```python
from build123d import *

# Parameters (mm, degrees)
BOSS_EXTRUDE1_DEPTH = 4
FILLET1_R           = 4
CHAMFER1_SIZE       = 3
CHAMFER2_SIZE       = 5
FILLET2_R           = 4
SKETCH2_R           = 1.6
CUT_EXTRUDE1_DEPTH  = 142.477913471
CUT_EXTRUDE2_DEPTH  = 2
FILLET3_R           = 3
SKETCH4_R           = 1.6
CUT_EXTRUDE3_DEPTH  = 142.477913471


with BuildPart() as part:
    # Sketch1 → Boss-Extrude1 (new body)
    with BuildSketch(Plane.XY):
        Polygon((-12, -87.8), (12, -87.8), (12, -56.4), (20, -56.4), (20, -95.8), (0, -115.8), (0, -140), (-20, -140), (-20, -95.8), align=None)
    extrude(amount=BOSS_EXTRUDE1_DEPTH)

    # Fillet1
    fillet1_edges = [part.edges().sort_by_distance(p)[0] for p in [
        (12, -56.4, 2),
        (20, -56.4, 2),
        (-20, -140, 2),
    ]]
    fillet(fillet1_edges, radius=FILLET1_R - 0.0001)  # a hair under: the kernel refuses the full size

    # Chamfer1
    chamfer1_edges = [part.edges().sort_by_distance(p)[0] for p in [
        (0, -140, 2),
    ]]
    chamfer(chamfer1_edges, length=CHAMFER1_SIZE)

    # Chamfer2
    chamfer2_edges = [part.edges().sort_by_distance(p)[0] for p in [
        (12, -87.8, 2),
    ]]
    chamfer(chamfer2_edges, length=CHAMFER2_SIZE)

    # Fillet2
    fillet2_edges = [part.edges().sort_by_distance(p)[0] for p in [
        (0, -115.8, 2),
        (20, -95.8, 2),
        (-12, -87.8, 2),
        (-20, -95.8, 2),
        (0, -137, 2),
        (-3, -140, 2),
        (7, -87.8, 2),
        (12, -82.8, 2),
    ]]
    fillet(fillet2_edges, radius=FILLET2_R)

    # Sketch2 → Cut-Extrude1 (cut, through all)
    with BuildSketch(Plane.XY.offset(4)):
        with Locations((0, -98.2)):
            Circle(SKETCH2_R)
    extrude(amount=-CUT_EXTRUDE1_DEPTH, mode=Mode.SUBTRACT)

    # Sketch3 → Cut-Extrude2 (cut)
    with BuildSketch(Plane.XY.offset(4)):
        Polygon((0, -129.942135624), (31.742135624, -98.2), (0, -66.457864376), (-31.742135624, -98.2), align=None)
    extrude(amount=-CUT_EXTRUDE2_DEPTH, mode=Mode.SUBTRACT)

    # Fillet3
    fillet3_edges = [part.edges().sort_by_distance(p)[0] for p in [
        (-20, -109.942135624, 3),
        (20, -86.457864376, 3),
        (12, -78.457864376, 3),
        (0, -129.942135624, 3),
    ]]
    fillet(fillet3_edges, radius=FILLET3_R)

    # Sketch4 → Cut-Extrude3 (cut, through all)
    with BuildSketch(Plane.XY.offset(4)):
        with Locations((-16, -136)):
            Circle(SKETCH4_R)
        with Locations((16, -60.4)):
            Circle(SKETCH4_R)
    extrude(amount=-CUT_EXTRUDE3_DEPTH, mode=Mode.SUBTRACT)


solid = part.part
```
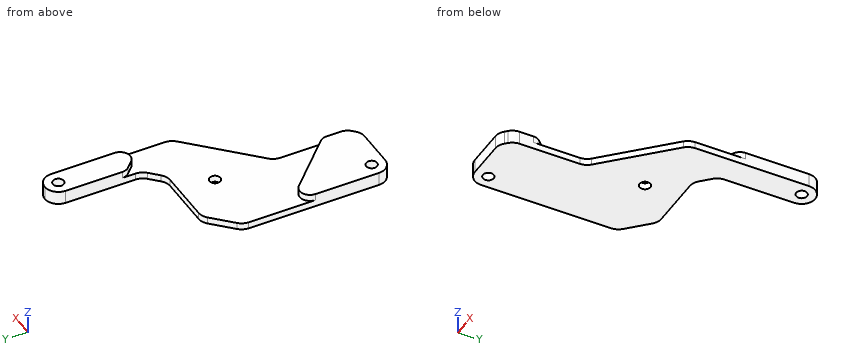
The model under review builds one solid part; all positions refer to its coordinate system, in mm. Round coordinates to 2 decimals unless told otherwise and drop trailing zeros. Order: outer loops, then holes, each group sorted by start corner. A loop starts at its lowest first (then second) coordinate and runs counter-clockwise, first axis right, second up. Notation, with made-up numbers: (-17, 22) -> (30, 22) arc R29 cw to (30, 58) -> close; hole circle Ø1 at (49, 45.5). An arc over 180 degrees is marked (long way). Use a Markdown table: item, result.
Q1. We need section C-C on y = -133. Write out the cut boundary in (x, z), then the cut area to 3 significant figures.
Values:
| item | result |
|---|---|
| outline | (-20, 0) -> (0, 0) -> (0, 4) -> (-20, 4) -> close |
| area | 80.0 mm^2 |
Q2. For line 1 (X direction, y = -98.2, z = 1.5); line 2 (Y direction, x = 16, z = 1.95); line 3 (Z direction, x = 5.5, y = -98.5), list the stretches that pass through material, from the lowest coordinate up.
Values:
| item | result |
|---|---|
| line 1 | x = -20 to -1.6, 1.6 to 17.6 |
| line 2 | y = -99.8 to -62, -58.8 to -56.4 |
| line 3 | z = 0 to 2 |
Q3. We need section B-B on y = -98.2. Write out the cut boundary in (x, z), then the cut area to 3 significant figures.
Values:
| item | result |
|---|---|
| outline | (-20, 0) -> (-1.6, 0) -> (-1.6, 2) -> (-20, 2) -> close; (1.6, 0) -> (17.6, 0) -> (17.6, 2) -> (1.6, 2) -> close |
| area | 68.8 mm^2 |
Q4. We need section A-A on z = 3.1. State how many separate pieces and enclosed holes the cut face has, then the cut area to 3 significant figures.
Values:
| item | result |
|---|---|
| separate pieces | 2 |
| enclosed holes | 2 |
| area | 555 mm^2 |
Q5. Clearance check with flat-ended pins moving along their axes: P1, Ø0.6, axis at x = -0.5, z = 1.5, coming from the +Y side; P2, Ø3, axis at x = 0, y = -98.2, coming from the -Z side; P3, Ø12, axis at x = -10.5, y = -103, coming from the +Z side; P4, Ø2, axis at y = -70, z = 2, coming from the -X side. State where each tip first meets the part, or that it passes through.
Values:
| item | result |
|---|---|
| P1 | stops at y = -87.8 |
| P2 | passes through |
| P3 | stops at z = 2 |
| P4 | stops at x = 12 |
Q6. We need section D-D on y = -121. Write out the cut boundary in (x, z).
Values:
| item | result |
|---|---|
| outline | (-20, 0) -> (0, 0) -> (0, 2) -> (-8.94, 2) -> (-8.94, 4) -> (-20, 4) -> close |
